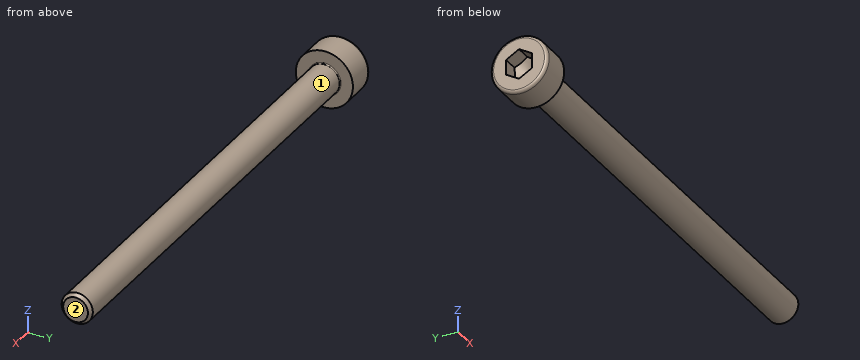
Autodesk Inventor part; units mm, degrees
ref_plane "Work Plane1" through (29, 0, 0) normal (0, -1, 0) x (1, 0, 0)
ref_plane "YZ Plane" through (0, 0, 0) normal (1, 0, 0) x (0, 1, 0)
ref_plane "XZ Plane" through (0, 0, 0) normal (0, 1, 0) x (-1, 0, 0)
sketch "Sketch1" plane through (0, 0, 0) normal (0, 0, 1) x (1, 0, 0)
  line L0 (-0.6667, 0) -> (45, 0)
  line L1 (45, 0) -> (45, 1.5)
  line L2 (45, 1.5) -> (27, 1.5)
  line L3 (27, 1.5) -> (26.6932, 1.5)
  line L4 (26.6932, 1.5) -> (0, 1.5)
  line L5 (0, 1.5) -> (0, 2.75)
  line L6 (0, 2.75) -> (-3, 2.75)
  line L7 (-3, 2.75) -> (-3, 1.4434)
  line L8 (-3, 1.4434) -> (-1.5, 1.4434)
  line L9 (-1.5, 1.4434) -> (-0.6667, 0)
  line L10 (-10.6, 0) -> (42.6, 0)
  line L11 (0, -0.55) -> (0, 3.3)
  line L12 (27, 1.5) -> (0, 1.5) construction
  dimension "d1" = 18
  dimension "d2" = 0.3068
  dimension "d3" = 3
  dimension "d4" = 1.5
  dimension "d5" = 60
  dimension "d6" = 3
  dimension "d7" = 3
  dimension "d8" = 2.8868
  dimension "d9" = 5.5
  dimension "d26" = 45
revolve "Body" add sketch "Sketch1" angle 360 about axis through (-0.6667, 0, 0) along (1, 0, 0)
sketch "Sketch2" plane through (-3, 0, 0) normal (-1, 0, 0) x (0, 0, 1)
  circle A0 centre (0, 0) radius 1.4434
  line L0 (0, -3.85) -> (0, 3.85)
  line L1 (-3.85, 0) -> (3.85, 0)
  line L2 (1.4434, 0) -> (0.7217, -1.25)
  line L3 (0.7217, -1.25) -> (-0.7217, -1.25)
  line L4 (-0.7217, -1.25) -> (-1.4434, 0)
  line L5 (-1.4434, 0) -> (-0.7217, 1.25)
  line L6 (-0.7217, 1.25) -> (0.7217, 1.25)
  line L7 (0.7217, 1.25) -> (1.4434, 0)
  point P0 (0, 0)
extrude "Slot" add sketch "Sketch2" against normal up to next contours L7 A0 | A0 L2 | L6 L0 A0 | A0 L0 L3 | L0 L6 A0 | A0 L3 L0 | L4 A0 | A0 L5
fillet "Fillet1" radius 0.3 1 edges at (-3, -2.75, 0)
thread "Thread"
chamfer "Chamfer1" distance 0.3067 distance2 0.3067 1 edges at (45, -1.5, 0) measured on face at (45, -0.8088, -0.4964)
ref_plane "Work Plane1" through (29, 0, 0) normal (0, -1, 0) x (1, 0, 0)
fillet "Fillet2" radius 0.1 1 edges at (0, -1.5, 0)
equation "\"d1\" = GEL"
equation "\"d3\" = KOH"
equation "\"d4\" = INTI"
equation "\"d6\" = GD"
equation "\"d7\" = BDM"
equation "\"d8\" = 1.1547 * SW"
equation "\"d9\" = KOD"
equation "\"d26\" = NLG"
equation "\"d30\" = R"
equation "\"d17\" = RR"
equation "\"d13\" = GEL"
equation "\"d15\" = -0.5 * SPD + 0.5 * GD"
equation "\"d16\" = GUL"
equation "\"GD\" = NND"
equation "\"NLG\" = 45"
equation "\"GEL\" = 18"
equation "\"KOD\" = 5.5"
equation "\"KOH\" = 3"
equation "\"INTI\" = 1.5"
equation "\"GAL\" = 0.61345 * PTC"
equation "\"GUL\" = 0.61345 * PTC"
equation "\"BDM\" = NND"
equation "\"SW\" = 2.5"
equation "\"RR\" = 0.3"
equation "\"SPD\" = 2.38655"
equation "\"R\" = 0.1"
equation "\"TOA\" = 30deg"
equation "\"THREADDIA\" = 3"
equation "\"PTC\" = 0.5"
equation "\"NND\" = 3"
equation "\"E0\" = 1.155 * SW"
equation "\"GD1\" = THREADDIA - 1.2269 * PTC"
properties part number "M3x45" material "Steel, Mild"
Design review of the part built by this model. Coordinates are the model's own, in mm. Face numbers are marked on the shaded views. A direction names the side the tool comes from. Coordinates: 2 decimals unless noted, no trailing zeros. Order: outer loops, then holes, each group sorted by start corner. A loop starts at its lowest first (then second) coordinate and runs counter-clockwise, first axis right, second up. Notation, with made-up numbers: M 58,30.5 L 64,30.5 A25 cw 64,57.5 Z; hole C 14.25,40 d1. An arc over 180 degrees is marked long. Use a Markdown table: item, result.
(1) For the marked faces 1 and 2, list the 3-axis set-ups (+Z, -Z, +X, -X, +Y, -Y) from which the entire face can be reached by the end or side of a thin tool; tool diameter is ignored.
Worked answers:
| item | result |
|---|---|
| face 1 | +X |
| face 2 | +Z, -Z, +X, +Y, -Y |
(2) Add section A-A (x = 10). Give the boundary of the cut face in (y, z), then the cut area to 3 significant figures.
Worked answers:
| item | result |
|---|---|
| outline | C 0,0 d3 |
| area | 7.07 mm2 |
(3) Wall thickness on probe 1 along X at (y, z) = (-0.5, 2); probe 2 along Z at (x, y) = (31.5, 0.1); probe 3 along Z at (x, y) = (14, 0.6): over which ranges is each line inside the solid? List them lowest first.
Worked answers:
| item | result |
|---|---|
| probe 1 | x = -3 to 0 |
| probe 2 | z = -1.5 to 1.5 |
| probe 3 | z = -1.37 to 1.37 |
(4) For P1, Ø2, axis at x = 37, z = 0, coming from the -Y side; P2, Ø1, axis at x = 7, y = -1, coming from the +Z side; P3, Ø3, axis at x = 25, z = -0.5, coming from the +Y side, all flat-tipped, find the tip position at first contact; note any pin that passes through.
Worked answers:
| item | result |
|---|---|
| P1 | stops at y = -1.5 |
| P2 | stops at z = 1.41 |
| P3 | stops at y = 1.5 |
